from build123d import *

# Parameters (mm, degrees)
F0_W          = 141
F0_H          = 17
F0_W_2        = 20
F0_H_2        = 20
F0_H_3        = 2.5
F8_DEPTH      = 3
F1_DEPTH      = 20
F9_R          = 2.3
F10_DEPTH     = 3
F2_R          = 2.3
F3_DEPTH      = 164.001
F3_DEPTH_BACK = 23.001
F4_R          = 2.3
F5_DEPTH      = 3
F6_SIZE       = 3
F7_R          = 2


with BuildPart() as f8:
    # F0 (on Top) → F8 (new body)
    with BuildSketch(Plane.XY):
        with Locations((0, 1.5)):
            Rectangle(F0_W, F0_H)
        Polygon((-73.5, -10), (73.5, -10), (73.5, 10), (70.5, 10), (70.5, -7), (-70.5, -7), (-70.5, 10), (-73.5, 10), align=None)
        with Locations((-83.5, 0)):
            Rectangle(F0_W_2, F0_H_2)
        Polygon((-93.5, 10), (-73.5, 10), (-70.5, 10), (-70.5, 12.5), (-93.5, 12.5), align=None)
        with Locations((83.5, 0)):
            Rectangle(F0_W_2, F0_H_2)
        Polygon((73.5, 10), (93.5, 10), (93.5, 12.5), (70.5, 12.5), (70.5, 10), align=None)
        with Locations((0, 11.25)):
            Rectangle(F0_W, F0_H_3)
    extrude(amount=-F8_DEPTH)

    # F0 (on Top) → F1 (join)
    with BuildSketch(Plane.XY):
        Polygon((-73.5, -10), (73.5, -10), (73.5, 10), (70.5, 10), (70.5, -7), (-70.5, -7), (-70.5, 10), (-73.5, 10), align=None)
        Polygon((-93.5, 10), (-73.5, 10), (-70.5, 10), (-70.5, 12.5), (-93.5, 12.5), align=None)
        Polygon((73.5, 10), (93.5, 10), (93.5, 12.5), (70.5, 12.5), (70.5, 10), align=None)
    extrude(amount=F1_DEPTH)

    # F9 (on face) → F10 (cut, through all)
    with BuildSketch(Plane(origin=(0, 0, -3), x_dir=(1, 0, 0), z_dir=(0, 0, -1))):
        with Locations((-83.5, 0)):
            Circle(F9_R)
        with Locations((83.5, 0)):
            Circle(F9_R)
    extrude(amount=-F10_DEPTH, mode=Mode.SUBTRACT)

    # F2 (on face) → F3 (cut, two sides)
    with BuildSketch(Plane.YZ.offset(-70.5)) as f3_sk:
        with Locations((2, 10)):
            Circle(F2_R)
    extrude(amount=F3_DEPTH, mode=Mode.SUBTRACT)
    extrude(f3_sk.sketch, amount=-F3_DEPTH_BACK, mode=Mode.SUBTRACT)

    # F4 (on face) → F5 (cut, through all)
    with BuildSketch(Plane.XZ.offset(10)):
        with Locations((-58.5, 10)):
            Circle(F4_R)
        with Locations((58.5, 10)):
            Circle(F4_R)
    extrude(amount=-F5_DEPTH, mode=Mode.SUBTRACT)

    # F6
    f6_edges = [f8.edges().sort_by_distance(p)[0] for p in [
        (70.5, -7, 10),
        (70.5, 2.75, 0),
        (-70.5, -7, 10),
        (-70.5, 2.75, 0),
        (0, -7, 0),
    ]]
    chamfer(f6_edges, length=F6_SIZE)

    # F7
    f7_edges = [f8.edges().sort_by_distance(p)[0] for p in [
        (-93.5, 12.5, 8.5),
        (-70.5, 12.5, 11.5),
        (0, 12.5, -3),
        (-82, 12.5, 20),
        (82, 12.5, 20),
        (93.5, 12.5, 8.5),
        (70.5, 12.5, 11.5),
        (93.5, 1.25, -3),
        (-93.5, 1.25, -3),
        (-70.5, 4.25, 20),
        (70.5, 4.25, 20),
    ]]
    fillet(f7_edges, radius=F7_R)


solid = f8.part
Read the model definition and answer for the solid it produces. Units are mm, in the model's axes. A direction names the side the tool comes from. Round coordinates to 2 decimals unless told otherwise and drop trailing zeros. Order: outer loops, then holes, each group sorted by start corner. A loop starts at its lowest first (then second) coordinate and runs counter-clockwise, first axis right, second up.
1) The part is cut by section A-A on x = 58.5. Write down the section's boundary in (y, z), plus the area to 3 significant figures.
2) Flat-ended cylindrical pins translate along their axes: pin 1 (6 mm diameter, centred on x = 87, z = 10.5, fed in from -Y); pin 2 (8 mm diameter, centred on y = 7, z = 9, fed in from -X); pin 3 (6 mm diameter, centred on y = -2, z = 14.5, fed in from +X); pin 4 (5 mm diameter, centred on x = 33, z = 12, fed in from +Y). Find the tip coordinate at first contact, or state that the pin passes through.
3) The mould has two halves that part along X. Classify faces 6 (the face through (-68.448, -4.906, 1.854)), 7 (the face through (-93.5, 10.2, 4.9)), 8 (the face through (0.4, 12.5, -0.7)): released by +X, released by -X, zero draft, split by the parting line, or undercut.
4) The part is cut by section B-B on z = 10. Give the number of separate pieces and of enclosed holes in the cut face, plus the area to 3 significant figures.
5) Straight lines are drawn through the part: L1, parallel to X at y = 0, z = -1.3; L2, parallel to X at y = 4, z = 4.75; L3, parallel to Z at x = -72.75, y = 2. For each, find the intervals that lie inside material, in ascending order.
6) For faces 1 (the face through (81.202, -0.101, -1.521)), 2 (the face through (-71.98, 1.7, 12.28)), 3 (the face through (73.5, -2, 10)), 4 (the face through (-84, 10, 10)), 5 (the face through (68.9, 4.4, 1.4)), determine the directions among +Z, -Z, +X, -X, +Y, -Y from which every point of the face is accessible in a straight line to the end or side of a thin tool.
7) The part is cut by section D-D on x = 26. Write down the section's boundary in (y, z), plus the area to 3 significant figures.
8) The part is cut by section C-C on y = 8. Write down the section's boundary in (x, z), plus the area to 3 significant figures.
Resolved:
1. outline: (-10, -3) - (10.5, -3) arc R2 ccw to (12.5, -1) - (12.5, 0) - (-4, 0) - (-7, 3) - (-7, 7.7) - (-10, 7.7) - close; (-10, 12.3) - (-7, 12.3) - (-7, 20) - (-10, 20) - close
1. area: 117 mm2
2. pin 1: stops at y = 10
2. pin 2: stops at x = -93.5
2. pin 3: stops at x = 73.5
2. pin 4: stops at y = -7
3. face 6: undercut
3. face 7: released by -X
3. face 8: zero draft
4. separate pieces: 5
4. enclosed holes: 0
4. area: 608 mm2
5. L1: x = -93.48 to -85.8, -81.2 to 81.2, 85.8 to 93.48
5. L2: x = -73.5 to -70.5, 70.5 to 73.5
5. L3: z = -3 to 7.7, 12.3 to 20
6. face 1: +Z, -Z
6. face 2: +X, -X
6. face 3: +Z, +X, -Y
6. face 4: +Z, -X, -Y
6. face 5: +Z, +Y
7. outline: (-10, -3) - (10.5, -3) arc R2 ccw to (12.5, -1) - (12.5, 0) - (-4, 0) - (-7, 3) - (-7, 20) - (-10, 20) - close
7. area: 131 mm2
8. outline: (-93.5, -1) arc R2 ccw to (-91.5, -3) - (91.5, -3) arc R2 ccw to (93.5, -1) - (93.5, 0) - (73.5, 0) - (73.5, 20) - (72.5, 20) arc R2 ccw to (70.5, 18) - (70.5, 3) - (67.5, 0) - (-67.5, 0) - (-70.5, 3) - (-70.5, 18) arc R2 ccw to (-72.5, 20) - (-73.5, 20) - (-73.5, 0) - (-93.5, 0) - close
8. area: 687 mm2
